from build123d import *

# Parameters (mm, degrees)
CROQUIS1_R              = 4
SALIENTE_EXTRUIR1_DEPTH = 1.7


with BuildPart() as part:
    # Croquis1 → Saliente-Extruir1 (new body)
    with BuildSketch(Plane.XY):
        with BuildLine():
            Line((-7, 25), (-7, 0))
            ThreePointArc((-7, 0), (0, -7), (7, 0))
            Line((7, 0), (7, 25))
            ThreePointArc((7, 25), (0, 32), (-7, 25))
        make_face()
        Circle(CROQUIS1_R, mode=Mode.SUBTRACT)
        with BuildLine():
            ThreePointArc((4, 25), (0, 29), (-4, 25))
            ThreePointArc((-4, 25), (0, 21), (4, 25))
        make_face(mode=Mode.SUBTRACT)
    extrude(amount=SALIENTE_EXTRUIR1_DEPTH)


solid = part.part
Work out the finished part from the listing and answer in its coordinate system (mm). Round coordinates to 2 decimals unless told otherwise and drop trailing zeros. Write each loop counter-clockwise with the first axis right and the second up, starting at its lowest first coordinate (ties: lowest second). Pieces come first, ordered by that corner, then holes.
1) The mould has two halves that part along Y. Classify faces 1 (the cylindrical face through (-0.867, -3.905, 0.838)), 2 (the flat face through (0, 13, 1.7)), 3 (the cylindrical face through (0.521, 21.034, 0.838)), 4 (the cylindrical face through (0, 32, 1)): pulls with the +Y half, pulls with the -Y half, needs draft (parallel to the pull), parting line crosses it, or undercut.
2) A cutting plane is placed at C-C (z = 0.9). Give the vertices of the cut face in (x, y).
3) A cutting plane is placed at A-A (x = 0). Give the vertices of the cut face in (y, z), plus the area to 3 significant figures.
4) A cutting plane is placed at D-D (x = 3.5). Give the vertices of the cut face in (y, z), plus the area to 3 significant figures.
5) Straight lines are drawn through the part: line 1 (Y direction, x = 0, z = 1.25); line 2 (Y direction, x = -2, z = 0.95); line 3 (X direction, y = 25, z = 0.5). For each, find the intervals that lie inside material, in ascending order.
6) A cutting plane is placed at B-B (y = -3). Give the vertices of the cut face in (x, z), plus the area to 3 significant figures.
Completed:
1. face 1: undercut
1. face 2: needs draft
1. face 3: undercut
1. face 4: pulls with the +Y half
2. outline: (-7, 0) arc R7 ccw to (7, 0) - (7, 25) arc R7 ccw to (-7, 25) - close; hole circle Ø8 at (0, 0); hole circle Ø8 at (0, 25)
3. outline: (-7, 0) - (-4, 0) - (-4, 1.7) - (-7, 1.7) - close; (4, 0) - (21, 0) - (21, 1.7) - (4, 1.7) - close; (29, 0) - (32, 0) - (32, 1.7) - (29, 1.7) - close
3. area: 39.1 mm2
4. outline: (-6.06, 0) - (-1.94, 0) - (-1.94, 1.7) - (-6.06, 1.7) - close; (1.94, 0) - (23.06, 0) - (23.06, 1.7) - (1.94, 1.7) - close; (26.94, 0) - (31.06, 0) - (31.06, 1.7) - (26.94, 1.7) - close
4. area: 49.9 mm2
5. line 1: y = -7 to -4, 4 to 21, 29 to 32
5. line 2: y = -6.71 to -3.46, 3.46 to 21.54, 28.46 to 31.71
5. line 3: x = -7 to -4, 4 to 7
6. outline: (-6.32, 0) - (-2.65, 0) - (-2.65, 1.7) - (-6.32, 1.7) - close; (2.65, 0) - (6.32, 0) - (6.32, 1.7) - (2.65, 1.7) - close
6. area: 12.5 mm2
